```python
from build123d import *

# Parameters (mm, degrees)
SKETCH_1_W          = 81
SKETCH_1_H          = 30
EXTRUDE_1_DEPTH     = 4
SKETCH_2_W          = 3
SKETCH_2_H          = 30
EXTRUDE_2_DEPTH     = 20
CUT_EXTRUDE_1_REACH = 90.662
SKETCH_3_R          = 1.5
SKETCH_4_W          = 3
SKETCH_4_H          = 30
EXTRUDE_3_DEPTH     = 30
CUT_EXTRUDE_2_REACH = 86.244
CUT_EXTRUDE_3_REACH = 86.244
SKETCH_8_R          = 1.5
SKETCH_9_W          = 68
SKETCH_9_H          = 54
CUT_EXTRUDE_4_DEPTH = 30


with BuildPart() as part:
    # 草图1 → 凸台-拉伸1 (new body)
    with BuildSketch(Plane.XY):
        with Locations((40.5, -15)):
            Rectangle(SKETCH_1_W, SKETCH_1_H)
    extrude(amount=EXTRUDE_1_DEPTH)

    # 草图2 → 凸台-拉伸2 (add)
    with BuildSketch(Plane(origin=(0, 0, 0), x_dir=(-1, 0, 0), z_dir=(0, 0, -1))):
        with Locations((-1.5, -15)):
            Rectangle(SKETCH_2_W, SKETCH_2_H)
        with Locations((-79.5, -15)):
            Rectangle(SKETCH_2_W, SKETCH_2_H)
    extrude(amount=EXTRUDE_2_DEPTH)

    # 切除-拉伸1: up to this face of the body (flat: up to its plane)
    cut_extrude_1_end = Plane(part.part.faces().sort_by_distance((81, -15, -8))[0])
    # 草图3 → 切除-拉伸1 (cut, up to the picked face)
    with BuildSketch(Plane.ZY, mode=Mode.PRIVATE) as cut_extrude_1_sk1:
        with Locations((-10, -15)):
            Circle(SKETCH_3_R)
    cut_extrude_1_tool1 = split(extrude(cut_extrude_1_sk1.sketch, amount=-CUT_EXTRUDE_1_REACH, mode=Mode.PRIVATE), bisect_by=cut_extrude_1_end, keep=Keep.BOTH, mode=Mode.PRIVATE)
    add(cut_extrude_1_tool1.solids().sort_by(Axis((0, -15, -10), (1, 0, 0)))[0], mode=Mode.SUBTRACT)

    # 草图4 → 凸台-拉伸3 (add)
    with BuildSketch(Plane.XY.offset(4)):
        with Locations((11.5, -15)):
            Rectangle(SKETCH_4_W, SKETCH_4_H)
        with Locations((69.5, -15)):
            Rectangle(SKETCH_4_W, SKETCH_4_H)
    extrude(amount=EXTRUDE_3_DEPTH)

    # 切除-拉伸2: up to this face of the body (flat: up to its plane)
    cut_extrude_2_end = Plane(part.part.faces().sort_by_distance((71, -15, 19))[0])
    # 草图7 → 切除-拉伸2 (cut, up to the picked face)
    with BuildSketch(Plane.ZY.offset(-10), mode=Mode.PRIVATE) as cut_extrude_2_sk1:
        with BuildLine():
            Line((34, 0), (19, 0))
            ThreePointArc((19, 0), (29.606601718, -4.393398282), (34, -15))
            Line((34, -15), (34, 0))
        make_face()
    cut_extrude_2_tool1 = split(extrude(cut_extrude_2_sk1.sketch, amount=-CUT_EXTRUDE_2_REACH, mode=Mode.PRIVATE), bisect_by=cut_extrude_2_end, keep=Keep.BOTH, mode=Mode.PRIVATE)
    # 草图7 → 切除-拉伸2 (cut, up to the picked face)
    with BuildSketch(Plane.ZY.offset(-10), mode=Mode.PRIVATE) as cut_extrude_2_sk2:
        with BuildLine():
            ThreePointArc((34, -15), (29.606601718, -25.606601718), (19, -30))
            Line((19, -30), (34, -30))
            Line((34, -30), (34, -15))
        make_face()
    cut_extrude_2_tool2 = split(extrude(cut_extrude_2_sk2.sketch, amount=-CUT_EXTRUDE_2_REACH, mode=Mode.PRIVATE), bisect_by=cut_extrude_2_end, keep=Keep.BOTH, mode=Mode.PRIVATE)
    add(cut_extrude_2_tool1.solids().sort_by(Axis((10, -3.350519, 30.649481), (1, 0, 0)))[0], mode=Mode.SUBTRACT)
    add(cut_extrude_2_tool2.solids().sort_by(Axis((10, -26.649481, 30.649481), (1, 0, 0)))[0], mode=Mode.SUBTRACT)

    # 切除-拉伸3: up to this face of the body (flat: up to its plane)
    cut_extrude_3_end = Plane(part.part.faces().sort_by_distance((71, -15, 17.599752116))[0])
    # 草图8 → 切除-拉伸3 (cut, up to the picked face)
    with BuildSketch(Plane.ZY.offset(-10), mode=Mode.PRIVATE) as cut_extrude_3_sk1:
        with Locations((19, -15)):
            Circle(SKETCH_8_R)
    cut_extrude_3_tool1 = split(extrude(cut_extrude_3_sk1.sketch, amount=-CUT_EXTRUDE_3_REACH, mode=Mode.PRIVATE), bisect_by=cut_extrude_3_end, keep=Keep.BOTH, mode=Mode.PRIVATE)
    add(cut_extrude_3_tool1.solids().sort_by(Axis((10, -15, 19), (1, 0, 0)))[0], mode=Mode.SUBTRACT)

    # 草图9 → 切除-拉伸4 (cut)
    with BuildSketch(Plane.XZ.offset(30)):
        with Locations((47, 7)):
            Rectangle(SKETCH_9_W, SKETCH_9_H)
    extrude(amount=-CUT_EXTRUDE_4_DEPTH, mode=Mode.SUBTRACT)


solid = part.part
```
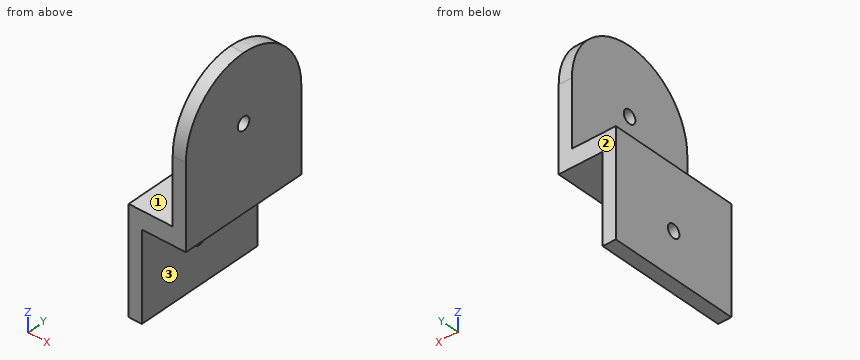
For this review, take the finished solid that the model builds, in its own axes (mm). Face numbers are marked on the shaded views. A direction names the side the tool comes from. Coordinates: 2 decimals unless noted, no trailing zeros. Order: outer loops, then holes, each group sorted by start corner. A loop starts at its lowest first (then second) coordinate and runs counter-clockwise, first axis right, second up. Notation, with made-up numbers: (63, 27.5) -> (86, 27.5) arc R8 ccw to (86, 34.5) -> close; hole circle Ø9 at (-13.5, 28.5). An arc over 180 degrees is marked (long way). Use CSV: the item, a comma, the result in double quotes. Start each with the question number.
Item 1: We need section C-C, the plane y = -23.5. Give the boundary of the cut face in (x, z).
Item 2: Wall thickness on probe 1 along Y at (x, z) = (0.85, -10); probe 2 along X at (y, z) = (-12, -17); probe 3 along X at (y, z) = (-19.75, 15): over which ranges is each line inside the solid? List them lowest first.
Item 3: For the marked faces 1, 2 and 3, list the 3-axis set-ups (+Z, -Z, +X, -X, +Y, -Y) from which the entire face can be reached by the end or side of a thin tool; tool diameter is ignored.
Item 4: We need section A-A, the plane x = 1.25. Give the boundary of the cut face in (y, z).
Item 5: Insertion check: pin 1 (1 mm diameter, centred on y = -5.5, z = 13, fed in from -X); pin 2 (5 mm diameter, centred on x = 6, z = -11, fed in from +Y); pin 3 (6 mm diameter, centred on x = 7.5, y = -14, fed in from -Z); pin 4 (2 mm diameter, centred on x = 6.5, y = -26.5, fed in from +Z). Each pin has a flat end and moves straight along its axis. Give the tip position at first contact, or say it passes through.
Item 6: We need section B-B, the plane z = -10. Give the boundary of the cut face in (x, y).
Item 7: We need section D-D, the plane z = 12. Give the boundary of the cut face in (x, y).
Derived:
1,outline,"(0, -20) -> (3, -20) -> (3, 0) -> (13, 0) -> (13, 31.36) -> (10, 31.36) -> (10, 4) -> (0, 4) -> close"
2,probe 1,"y = -30 to -16.5, -13.5 to 0"
2,probe 2,"x = 0 to 3"
2,probe 3,"x = 10 to 13"
3,face 1,"+Z, -X, +Y, -Y"
3,face 2,"+Z, -Z, +X, -X, +Y"
3,face 3,"-Z, +X, +Y, -Y"
4,outline,"(-30, -20) -> (0, -20) -> (0, 4) -> (-30, 4) -> close; hole circle Ø3 at (-15, -10)"
5,pin 1,"stops at x = 10"
5,pin 2,"passes through"
5,pin 3,"stops at z = 0"
5,pin 4,"stops at z = 4"
6,outline,"(0, -30) -> (3, -30) -> (3, -16.5) -> (0, -16.5) -> close; (0, -13.5) -> (3, -13.5) -> (3, 0) -> (0, 0) -> close"
7,outline,"(10, -30) -> (13, -30) -> (13, 0) -> (10, 0) -> close"
